Autodesk Inventor part; units mm, degrees
ref_plane "YZ Plane" through (0, 0, 0) normal (1, 0, 0) x (0, 1, 0)
ref_plane "XZ Plane" through (0, 0, 0) normal (0, 1, 0) x (-1, 0, 0)
ref_plane "XY Plane" through (0, 0, 0) normal (0, 0, 1) x (1, 0, 0)
sketch "Sketch5" plane through (0, 0, 0) normal (0, 0, 1) x (1, 0, 0)
  line L0 (-10, -12.5) -> (10, -12.5)
  line L1 (10, -12.5) -> (10, 12.5)
  line L2 (10, 12.5) -> (-10, 12.5)
  line L3 (-10, 12.5) -> (-10, -12.5)
  line L4 (-10, -12.5) -> (10, 12.5) construction
  line L5 (10, -12.5) -> (-10, 12.5) construction
  circle A0 centre (15, 0) radius 1.5
  circle A1 centre (-15, 0) radius 1.5
  line L6 (-20, -15) -> (20, -15)
  line L7 (20, -15) -> (20, 15)
  line L8 (20, 15) -> (-20, 15)
  line L9 (-20, 15) -> (-20, -15)
  line L10 (-20, -15) -> (20, 15) construction
  line L11 (20, -15) -> (-20, 15) construction
  line L12 (-20, 0) -> (20, 0)
  line L13 (0, -15) -> (0, 15)
  point P0 (0, 0)
  dimension "d27" = 20
  dimension "d28" = 25
  dimension "d29" = 3
  dimension "d30" = 15
  dimension "d31" = 30
  dimension "d36" = 40
extrude "Extrusion4" add sketch "Sketch5" along normal blind 20 contours L0 L13 L6 L9 L12 A1 L3 | L0 L1 L12 A0 L7 L6 L13 | L12 A1 L9 L8 L13 L2 L3 | L1 L2 L13 L8 L7 L12 A0
extrude "Extrusion5" add sketch "Sketch5" along normal blind 5 contours L3 L12 L13 L0 | L13 L12 L1 L0 | L3 L2 L13 L12 | L13 L2 L1 L12
extrude "Extrusion6" add sketch "Sketch5" along normal blind 5 contours L12 A1 | A1 L12 | L12 A0 | A0 L12
fillet "Fillet3" radius 2 8 edges at (20, 0, 0) (20, 15, 10) (20, 0, 20) (20, -15, 10) (-20, 0, 0) (-20, -15, 10) (-20, 0, 20) (-20, 15, 10)
sketch "Sketch9" plane through (0, 0, 0) normal (1, 0, 0) x (0, 1, 0)
  line L0 (-12.5, 20) -> (12.5, 20)
  line L1 (-36, 20) -> (36, 20)
  arc A0 (36, 20) -> (38, 22) centre (36, 22) ccw
  line L2 (38, 22) -> (38, 23)
  line L3 (15, 0) -> (15, 20)
  line L4 (38, 23) -> (52.0954, 17.8697)
  line L5 (38, 23) -> (53, 23) construction
  line L6 (-15, 0) -> (-15, 20)
  line L7 (-15, 0) -> (-5, 0) construction
  line L8 (-15, 0) -> (15, 0)
  line L9 (15, 20) -> (15, 0)
  line L10 (-15, 0) -> (-15, 20)
  line L11 (-15, 20) -> (-20, 20)
  arc A1 (-15, 15) -> (-20, 20) centre (-20, 15) ccw
  line L12 (-20, 20) -> (-15, 15) construction
  line L13 (-20, 20) -> (-12.9289, 20) construction
  line L14 (-1.898, -79.3761) -> (19.3152, -100.5893)
  line L15 (19.3152, -100.5893) -> (31.7976, -97.2447)
  line L16 (52.0954, 17.8697) -> (31.7976, -97.2447)
  line L17 (-15, 0) -> (-7.0211, -23.6926)
  arc A2 (-7.0211, -23.6926) -> (-15, 0) centre (-29.9276, -18.217) ccw
  line L18 (-7.0211, -23.6926) -> (0.0266, -26.2577)
  line L19 (-7.0211, -23.6926) -> (0.4789, -23.6926) construction
  line L20 (0.0266, -26.2577) -> (-1.898, -79.3761)
  arc A3 (-0.9357, -52.8168) -> (0.0266, -26.2577) centre (-15.8648, -38.9789) ccw
  arc A4 (-1.898, -79.3761) -> (-0.9357, -52.8168) centre (-22.5407, -65.3311) ccw
  point P0 (0, 0)
  point P1 (0, 20)
  dimension "d46" = 72
  dimension "d47" = 2
  dimension "d48" = 1
  dimension "d60" = 15
  dimension "d61" = 20
  dimension "d73" = 5
  dimension "d74" = 45
  dimension "d79" = 30
  dimension "d81" = 120
  dimension "d91" = 25
  dimension "d94" = 7.5
  dimension "d95" = 20
  dimension "d96" = 26.5765
extrude "Extrusion10" add sketch "Sketch9" along normal mid plane 30 contours L6 A1 L1 | L1 A0 L2 L4 L16 L15 L14 A4 A3 L18 A2 L8 L3
fillet "Fillet4" radius 2 23 edges at (15, -7.6075, -10.7002) (0, 0.0266, -26.2577) (15, -3.4973, -24.9751) (0, -7.0211, -23.6926) (-15, -3.4973, -24.9751) (0, -1.898, -79.3761) (15, 2.4106, -66.2351) (0, -0.9357, -52.8168) (-15, 2.4106, -66.2351) (15, 4.4778, -39.716) (-15, 4.4778, -39.716) (0, 19.3152, -100.5893) (15, 8.7086, -89.9827) (-15, 8.7086, -89.9827) (0, 31.7976, -97.2447) (15, 25.5564, -98.917) (-15, 25.5564, -98.917) (-15, -7.6075, -10.7002) (0, 52.0954, 17.8697) (15, 41.9465, -39.6875) (-15, 41.9465, -39.6875) (-15, 45.0477, 20.4348) (15, 45.0477, 20.4348)
thread "Thread3"
thread "Thread4"
sketch "Sketch10" plane through (20, -13, 2) normal (1, 0, 0) x (0, 0, -1)
  line L0 (-16, 0) -> (-16, 26)
  line L1 (-16, 13) -> (-12, 13)
  line L2 (-12, 13) -> (-12, 17)
  line L3 (-12, 17) -> (-16, 17)
  line L4 (-16, 17) -> (-16, 13)
  line L5 (-16, 13) -> (-12, 13)
  line L6 (-12, 13) -> (-12, 9)
  line L7 (-12, 9) -> (-16, 9)
  line L8 (-16, 9) -> (-16, 13)
  point P0 (2, 13)
  dimension "d104" = 4
  dimension "d105" = 4
  dimension "d106" = 4
extrude "Extrusion11" cut sketch "Sketch10" against normal through all
properties part number "Controller Handle"
Input: part model. Units: mm. Frame: model coordinates. A direction names the side the tool comes from. Coordinates: 2 decimals unless noted, no trailing zeros.
Q1. Draft query along Y for faces 1 (the face through (-14.43, 44.141, 20.125)), 2 (the face through (-0.182, -7.946, -9.761)), 3 (the face through (-15, 25, -38)), 4 (the face through (-10, 0, 12)). Return one class per face: +Y half, -Y half, draft (parallel to the pull), parting line (faces both ways), or undercut.
Q2. Material intervals for line 1 (X direction, y = 0, z = 9); line 2 (X direction, y = -5.5, z = -17); line 3 (X direction, y = 0, z = 18.85), sorted ascending.
Q3. Contact query for flat-ended pins moving along their axis: pin 1 (5 mm diameter, centred on x = 15, y = 0, fed in from +Z); pin 2 (8 mm diameter, centred on x = 3.5, y = 1.5, fed in from -Z); pin 3 (18.5 mm diameter, centred on y = 33, z = -53, fed in from -X). Output: stop coordinate, or through.
Q4. Set-up query: faces 5 (the face through (-14.4, 25.42, -98.36)), 6 (the face through (10, 0, 12)), 7 (the face through (-15, 2, 14)). Return all of +Z, -Z, +X, -X, +Y, -Y with unobstructed straight access to the full face (end or side cutting, diameter ignored); none if empty.
Working result:
1. face 1: +Y half
1. face 2: -Y half
1. face 3: draft
1. face 4: undercut
2. line 1: x = -20 to -16.5, -13.5 to -10, 10 to 13.5, 16.5 to 20
2. line 2: x = -14.67 to 14.67
2. line 3: x = -19.81 to -16.5, -13.5 to -10, 10 to 13.5, 16.5 to 19.81
3. pin 1: stops at z = 20
3. pin 2: stops at z = -86.77
3. pin 3: stops at x = -15
4. face 5: -Z, -X, +Y
4. face 6: +Z
4. face 7: +X, -X
